```python
from build123d import *

# Parameters (mm, degrees)
F0_W     = 177.8
F0_H     = 177.8
F1_DEPTH = 50.8
F2_DEPTH = 25.4
F3_W     = 50.8
F3_H     = 76.2
F4_DEPTH = 50.8


# Not quite as in the source:
# - a feature names something its author has since deleted; it is built from what else it names


with BuildPart() as f1:
    # F0 (on Front) → F1 (new body)
    with BuildSketch(Plane.XZ):
        with Locations((0.9207129478, 25.5247855931)):
            Rectangle(F0_W, F0_H)
    extrude(amount=F1_DEPTH)

    # F2 (add, symmetric): a face of the model
    f2_faces = [f1.faces().sort_by_distance(p)[0] for p in [
        (0.9207129478, -50.8, 25.5247855931),
    ]]
    extrude(f2_faces, amount=F2_DEPTH, both=True)

    # F3 (on face) → F4 (join)
    with BuildSketch(Plane.XZ.offset(76.2)):
        with Locations((-62.5792870522, 76.3247855931)):
            Rectangle(F3_W, F3_H)
        with Locations((64.4207129478, 76.3247855931)):
            Rectangle(F3_W, F3_H)
    extrude(amount=F4_DEPTH)


solid = f1.part
```
Model file for the job. Use its own axes, mm. A direction names the side the tool comes from. Round coordinates to 2 decimals unless told otherwise and drop trailing zeros. Write each loop counter-clockwise with the first axis right and the second up, starting at its lowest first coordinate (ties: lowest second). Pieces come first, ordered by that corner, then holes. Notation, with made-up numbers: (-5, 85) - (8, 85) arc R29 ccw to (8, 118) - close; hole circle Ø2 at (5.5, 63). An arc over 180 degrees is marked (long way). Use CSV: the item, a comma, the result in double quotes. Start each with the question number.
Item 1: Band-saw the part on C-C (x = 64). Write the cut outline in (y, z).
Item 2: Band-saw the part on A-A (y = -99.5). Write the cut outline in (x, z).
Item 3: Band-saw the part on B-B (z = 61.5). Write the cut outline in (x, y).
Item 4: Band-saw the part on D-D (z = -12.5). Write the cut outline in (x, y), and give its area (3 significant figures).
Item 5: Tool access for faces 4 (the face through (39.021, -101, 76)), 5 (the face through (64, -127, 77)), 6 (the face through (-63, -101, 38.225)): list every direction of +Z, -Z, +X, -X, +Y, -Y with a clear straight run to the whole face (end or side of a thin tool).
Item 6: Drill centre lines: L1, parallel to X at y = -117.5, z = 68.5; L2, parallel to Y at x = -5, z = 53; L3, parallel to Z at x = 56, y = -86. Where is each one in solid material? Low to high. Write a range as [from, to].
Item 7: Pin check, flat tips, straight feed: P1, Ø15, axis at x = 67, y = -102, coming from the -Z side; P2, Ø10, axis at x = -60.5, z = -28, coming from the -Y side. Stop position of each tip, or through.
Item 8: Two-plate mould, pull along X, no slides. Class faces 1 (the face through (89.821, -48, 44)), 2 (the face through (64, -101, 38.225)), 3 (the face through (-37.179, -101, 76)): released by +X, released by -X, zero draft, split by the parting line, or undercut.
Checked values:
1,outline,"(-127, 38.22) - (-76.2, 38.22) - (-76.2, -63.38) - (0, -63.38) - (0, 114.42) - (-127, 114.42) - close"
2,outline,"(-87.98, 38.22) - (-37.18, 38.22) - (-37.18, 114.42) - (-87.98, 114.42) - close; (39.02, 38.22) - (89.82, 38.22) - (89.82, 114.42) - (39.02, 114.42) - close"
3,outline,"(-87.98, -127) - (-37.18, -127) - (-37.18, -76.2) - (39.02, -76.2) - (39.02, -127) - (89.82, -127) - (89.82, 0) - (-87.98, 0) - close"
4,outline,"(-87.98, -76.2) - (89.82, -76.2) - (89.82, 0) - (-87.98, 0) - close"
4,area,"13,500 mm²"
5,face 4,"+Z, -Z, -Y"
5,face 5,"+Z, -Z, +X, -X, -Y"
5,face 6,"-Z, +X, -X, -Y"
6,L1,"x = [-87.98, -37.18], [39.02, 89.82]"
6,L2,"y = [-76.2, 0]"
6,L3,"z = [38.22, 114.42]"
7,P1,"stops at z = 38.22"
7,P2,"stops at y = -76.2"
8,face 1,"released by +X"
8,face 2,"zero draft"
8,face 3,"undercut"
